from build123d import *

# Parameters (mm, degrees)
F0_W     = 10
F0_H     = 2
F1_DEPTH = 6
F2_W     = 22
F2_H     = 13.3
F3_DEPTH = 1


with BuildPart() as f1:
    # F0 (on Top) → F1 (new body)
    with BuildSketch(Plane.XY):
        Polygon((-5, 4.65), (5, 4.65), (5, 2.7), (7, 2.7), (7, 4.85), (7, 6.65), (5, 6.65), (-5, 6.65), align=None)
        with Locations((-10, 5.65)):
            Rectangle(F0_W, F0_H)
    extrude(amount=F1_DEPTH)



with BuildPart() as f1b:
    # F0 (on Top) → F1, piece 2 (new body)
    with BuildSketch(Plane.XY):
        Polygon((5, -4.65), (-5, -4.65), (-5, -6.65), (5, -6.65), (7, -6.65), (7, -4.85), (7, -2.7), (5, -2.7), align=None)
        with Locations((-10, -5.65)):
            Rectangle(F0_W, F0_H)
    extrude(amount=F1_DEPTH)


with BuildPart() as f1_1:
    add(f1.part)

    add(f1b.part)  # F3 merges F1b
    # F2 (on Top) → F3 (join)
    with BuildSketch(Plane.XY):
        with Locations((-4, 0)):
            Rectangle(F2_W, F2_H)
    extrude(amount=-F3_DEPTH)


solid = f1_1.part
Design review of the part built by this model. Coordinates are the model's own, in mm. A direction names the side the tool comes from. Round coordinates to 2 decimals unless told otherwise and drop trailing zeros. Order: outer loops, then holes, each group sorted by start corner. A loop starts at its lowest first (then second) coordinate and runs counter-clockwise, first axis right, second up.
1) Machinability: for faces 5 (the flat face through (6, -2.7, 3)), 6 (the flat face through (-5, 4.65, 3)), 7 (the flat face through (-4, 6, 6)), which of the approach directions +Z, -Z, +X, -X, +Y, -Y give a long, thin tool a straight path to every point of the face, cutting with its end or side? Answer none if there is none.
The answers:
face 5: +Z, +X, -X
face 6: +Z, -X
face 7: +Z, +X, -X, +Y, -Y
2) Draft analysis for pull direction Y (two halves, no side actions). For faces 1 (the flat face through (-4, -6.65, 3)), 2 (the flat face through (-4, 0, 0)), 3 (the flat face through (-15, 0.5, -0.3)), 4 (the flat face through (6, 2.7, 3)), state which applies: released by +Y, released by -Y, zero draft, split by the parting line, or undercut.
The answers:
face 1: released by -Y
face 2: undercut
face 3: zero draft
face 4: undercut
3) Consider section A-A (x = -11.25). State the section outline as (y, z) points, plus the area to 3 significant figures.
The answers:
outline: (-6.65, -1) - (6.65, -1) - (6.65, 6) - (4.65, 6) - (4.65, 0) - (-4.65, 0) - (-4.65, 6) - (-6.65, 6) - close
area: 37.3 mm2
4) Consider section B-B (z = 4). State the section outline as (x, y) points.
The answers:
outline: (-15, -6.65) - (7, -6.65) - (7, -2.7) - (5, -2.7) - (5, -4.65) - (-15, -4.65) - close; (-15, 4.65) - (5, 4.65) - (5, 2.7) - (7, 2.7) - (7, 6.65) - (-15, 6.65) - close
5) Clearance check with flat-ended pins moving along their axes: pin 1 Ø0.6 at (y, z) = (-4, 3.5) entering from -X; pin 2 Ø4.5 at (x, y) = (-2, -1.5) entering from +Z. State where each tip first meets the part, or that it passes through.
The answers:
pin 1: stops at x = 5
pin 2: stops at z = 0
6) For L1, parallel to Y at x = -1.5, z = 4; L2, parallel to X at y = -3, z = 3; L3, parallel to Z at x = 3, y = -0.75, list the stretches that pass through material, from the lowest coordinate up.
The answers:
L1: y = -6.65 to -4.65, 4.65 to 6.65
L2: x = 5 to 7
L3: z = -1 to 0
7) Consider section C-C (y = 0.75). State the section outline as (x, z) points.
The answers:
outline: (-15, -1) - (7, -1) - (7, 0) - (-15, 0) - close
